from build123d import *

# Parameters (mm, degrees)
SKETCH1_W             = 4.2
SKETCH1_H             = 9.05
BOSS_EXTRUDE1_DEPTH   = 150
M3X0_5_TAPPED_HOLE1_D = 2.5
LPATTERN1_COUNT       = 15
LPATTERN1_PITCH       = 20
SKETCH7_W             = 5.7
SKETCH7_H             = 2
BOSS_EXTRUDE3_DEPTH   = 300
SKETCH9_W             = 5.7
SKETCH9_H             = 3.05
CUT_EXTRUDE2_DEPTH    = 301


with BuildPart() as part:
    # Sketch1 → Boss-Extrude1 (new body, symmetric)
    with BuildSketch(Plane.XY):
        Rectangle(SKETCH1_W, SKETCH1_H)
    extrude(amount=BOSS_EXTRUDE1_DEPTH, both=True)

    # M3x0.5 Tapped Hole1 (through all)
    with Locations(Plane.ZY.offset(2.1)):
        with Locations((-140, 0)):
            m3x0_5_tapped_hole1 = Hole(M3X0_5_TAPPED_HOLE1_D / 2)

    # LPattern1: M3x0.5 Tapped Hole1 ×15
    with Locations(*[(0, 0, i * LPATTERN1_PITCH) for i in range(1, LPATTERN1_COUNT)]):
        add(m3x0_5_tapped_hole1, mode=Mode.SUBTRACT)

    # Sketch7 → Boss-Extrude3 (add)
    with BuildSketch(Plane.XY.offset(150)):
        with Locations((-0.75, 5.525)):
            Rectangle(SKETCH7_W, SKETCH7_H)
        with Locations((-0.75, -5.525)):
            Rectangle(SKETCH7_W, SKETCH7_H)
    extrude(amount=-BOSS_EXTRUDE3_DEPTH)

    # Sketch9 → Cut-Extrude2 (cut, through all)
    with BuildSketch(Plane.XY.offset(150)):
        with Locations((-0.75, 5)):
            Rectangle(SKETCH9_W, SKETCH9_H)
    extrude(amount=-CUT_EXTRUDE2_DEPTH, mode=Mode.SUBTRACT)


solid = part.part
Model file for the job. Use its own axes, mm. A direction names the side the tool comes from. Give positions to 0.01 mm unless a question says otherwise; leave off trailing zeros. Order: outer loops, then holes, each group sorted by start corner. A loop starts at its lowest first (then second) coordinate and runs counter-clockwise, first axis right, second up. Notation, with made-up numbers: M 27,36 L 71,36 A14 ccw 71,63 Z; hole C 60,1.25 d11. An arc over 180 degrees is marked long. Write item = value, one per line.
Q1. Cut at B-B, the plane z = -12. List the corners of the cut face in (x, y) (3 decimals), then the cut area to 3 significant figures.
Derived:
outline = M -3.6,-6.525 L 2.1,-6.525 L 2.1,3.475 L -2.1,3.475 L -2.1,-4.525 L -3.6,-4.525 Z
area = 45.0 mm2
Q2. Drill centre lines: line 1 (Y direction, x = -0.35, z = -60) (3 decimals); line 2 (X direction, y = -1.25, z = 81); line 3 (Y direction, x = -3.4, z = 108) (3 decimals). Where is each one in solid material? Low to high. Write a range as [from, to].
Derived:
line_1 = [-6.525, -1.25], [1.25, 3.475]
line_2 = [-2.1, 2.1]
line_3 = [-6.525, -4.525]
Q3. Tool access for faces 1 (the flat face through (-2.1, -1, 2)), 2 (the flat face through (0, -1, -150)): list every direction of +Z, -Z, +X, -X, +Y, -Y with a clear straight run to the whole face (end or side of a thin tool).
Derived:
face_1 = +Z, -Z, -X, +Y
face_2 = -Z, +X, -X, +Y, -Y
Q4. Flat gauge pins, fed straight in: pin 1 (2 mm diameter, centred on y = 0, z = 20, fed in from -X); pin 2 (3 mm diameter, centred on y = 0, z = -80, fed in from -X). Where does each tip first touch, or does it go through?
Derived:
pin_1 = through
pin_2 = -2.1
Q5. Cut at A-A, the plane x = 1.2. Count the separate pieces of the cut face and the enclosed holes in it, then the cut area to 3 significant figures.
Derived:
separate_pieces = 1
enclosed_holes = 15
area = 2,930 mm2
